```python
from build123d import *

# Parameters (mm, degrees)
BOX006_W                = 2
BOX006_H                = 4.17
BOX006_DEPTH            = 13
ARRAY003_X_COUNT        = 2
ARRAY003_X_PITCH        = 43
ARRAY003_Y_COUNT        = 2
ARRAY003_Y_PITCH        = 27.5
CYLINDER002_R           = 2.1
CYLINDER002_DEPTH       = 2
CYLINDER002_PITCH_ANGLE = 90
ARRAY002_X_COUNT        = 2
ARRAY002_X_PITCH        = 43
ARRAY002_Y_COUNT        = 2
ARRAY002_Y_PITCH        = 27.5
CYLINDER003_R           = 3.25
CYLINDER003_DEPTH       = 2
BOX007_W                = 6.5
BOX007_H                = 36
BOX007_DEPTH            = 2
BOX003_W                = 45
BOX003_H                = 60
BOX003_DEPTH            = 2
BOX005_W                = 2
BOX005_H                = 60
BOX005_DEPTH            = 45
BOX004_W                = 2
BOX004_H                = 60
BOX004_DEPTH            = 45
CUT003_PLACEMENT_ANGLE  = 180


with BuildPart() as array003:
    # Box006 → Box006 (new body)
    with BuildSketch(Plane(origin=(0, 15.6, 37), x_dir=(1, 0, 0), z_dir=(0, 0, 1))):
        with Locations((1, 2.085)):
            Rectangle(BOX006_W, BOX006_H)
    extrude(amount=BOX006_DEPTH)

    # Array003 X: Array003 ×2


with BuildPart() as array003_1:
    add(array003.part)
    with Locations(*[(i * ARRAY003_X_PITCH, 0, 0) for i in range(1, ARRAY003_X_COUNT)]):
        add(array003.part)

    # Array003 Y: Array003 ×2


with BuildPart() as array003_2:
    add(array003_1.part)
    with Locations(*[(0, i * ARRAY003_Y_PITCH, 0) for i in range(1, ARRAY003_Y_COUNT)]):
        add(array003_1.part)


with BuildPart() as fusion003:
    # Cylinder002 → Cylinder002 (new body)
    with BuildSketch(Plane.XY):
        Circle(CYLINDER002_R)
    extrude(amount=CYLINDER002_DEPTH)


with BuildPart() as fusion003_1:
    # Cylinder002 pitch: moved
    add(fusion003.part.rotate(Axis((0, 0, 0), (0, 1, 0)), CYLINDER002_PITCH_ANGLE))


with BuildPart() as fusion003_2:
    # Cylinder002 placement: moved
    add(fusion003_1.part.moved(Location((0, 17.7, 37.1))))

    # Array002 X: Fusion003 ×2


with BuildPart() as fusion003_3:
    add(fusion003_2.part)
    with Locations(*[(i * ARRAY002_X_PITCH, 0, 0) for i in range(1, ARRAY002_X_COUNT)]):
        add(fusion003_2.part)

    # Array002 Y: Fusion003 ×2


with BuildPart() as fusion003_4:
    add(fusion003_3.part)
    with Locations(*[(0, i * ARRAY002_Y_PITCH, 0) for i in range(1, ARRAY002_Y_COUNT)]):
        add(fusion003_3.part)

    # Fusion003: union Array003
    add(array003_2.part)


with BuildPart() as cilindro003:
    # Cylinder003 → Cylinder003 (new body)
    with BuildSketch(Plane(origin=(22.5, 30, 0), x_dir=(1, 0, 0), z_dir=(0, 0, 1))):
        Circle(CYLINDER003_R)
    extrude(amount=CYLINDER003_DEPTH)


with BuildPart() as fusion004:
    # Box007 → Box007 (new body)
    with BuildSketch(Plane(origin=(19.25, 30, 0), x_dir=(1, 0, 0), z_dir=(0, 0, 1))):
        with Locations((3.25, 18)):
            Rectangle(BOX007_W, BOX007_H)
    extrude(amount=BOX007_DEPTH)

    # Fusion002: union Cilindro003
    add(cilindro003.part)

    # Fusion004: union Fusion003
    add(fusion003_4.part)


with BuildPart() as pared_inferior:
    # Box003 → Box003 (new body)
    with BuildSketch(Plane.XY):
        with Locations((22.5, 30)):
            Rectangle(BOX003_W, BOX003_H)
    extrude(amount=BOX003_DEPTH)


with BuildPart() as pared_izquierda:
    # Box005 → Box005 (new body)
    with BuildSketch(Plane(origin=(43, 0, 0), x_dir=(1, 0, 0), z_dir=(0, 0, 1))):
        with Locations((1, 30)):
            Rectangle(BOX005_W, BOX005_H)
    extrude(amount=BOX005_DEPTH)


with BuildPart() as obj1:
    # Box004 → Box004 (new body)
    with BuildSketch(Plane.XY):
        with Locations((1, 30)):
            Rectangle(BOX004_W, BOX004_H)
    extrude(amount=BOX004_DEPTH)

    # Fusion001: union pared inferior, pared izquierda
    add(pared_inferior.part)
    add(pared_izquierda.part)

    # Cut003: cut Fusion004
    add(fusion004.part, mode=Mode.SUBTRACT)


with BuildPart() as obj1_1:
    # Cut003 placement: moved
    add(obj1.part.moved(Location((0, 12, 35))).rotate(Axis((0, 12, 35), (1, 0, 0)), CUT003_PLACEMENT_ANGLE))


solid = obj1_1.part
```
The listing builds one solid part. Answer for the finished solid, in the listing's coordinates (mm). A direction names the side the tool comes from. Round coordinates to 2 decimals unless told otherwise and drop trailing zeros. Loops run counter-clockwise (first coordinate to the right, second up) from the corner with the lowest first, then second, coordinate; pieces in that order, holes last. Notation, with made-up numbers: (-26.75, 40) - (12.25, 40) arc R20 cw to (12.25, 62) - close; hole circle Ø10 at (31, 45). An arc over 180 degrees is marked (long way). Return JSON: item names as keys, results as strings. Group by question number.
1. Each of these flat-tipped pins is pushed along its axis until it touches: P1, Ø12, axis at x = 29, y = -11.5, coming from the -Z side; P2, Ø6, axis at x = 6.5, z = 0, coming from the +Y side. Where does it stop, or does it pass through?
2. The mould has two halves that part along X. Classify faces 1 (the flat face through (17, -18, 35)), 2 (the flat face through (45, -18, 13)), 3 (the flat face through (2, -18, 12)), 4 (the flat face through (19.25, -33, 34)): pulls with the +X half, pulls with the -X half, needs draft (parallel to the pull), parting line crosses it, or undercut.
3. The part is cut by section A-A on y = -30. Determine the outline of the cut face in (x, z), then the cut area to 3 significant figures.
4. The part is cut by section D-D on x = 11. Determine the outline of the cut face in (y, z), then the cut area to 3 significant figures.
5. The part is cut by section C-C on y = -14. Determine the outline of the cut face in (x, z).
6. The part is cut by section B-B on z = 21. Determine the outline of the cut face in (x, y).
7. Which of the six approach directions +Z, -Z, +X, -X, +Y, -Y give full straight-line access (tool end or side, diameter ignored) to faces 5 (the flat face through (1, -7.77, -6)), 6 (the flat face through (22, 12, 34))?
8. Consider probe 1 along X at (y, z) = (-40.5, -3.5); probe 2 along Z at (x, y) = (10, -9). Determine where each line is inside the solid, lowest interval first.
Resolved:
{
 "1": {"P1": "stops at z = 33", "P2": "passes through"},
 "2": {"face 1": "needs draft", "face 2": "pulls with the +X half", "face 3": "undercut", "face 4": "undercut"},
 "3": {"outline": "(0, -10) - (2, -10) - (2, 33) - (19.25, 33) - (19.25, 35) - (0, 35) - close; (25.75, 33) - (43, 33) - (43, -10) - (45, -10) - (45, 35) - (25.75, 35) - close", "area": "249 mm²"},
 "4": {"outline": "(-48, 33) - (12, 33) - (12, 35) - (-48, 35) - close", "area": "120 mm²"},
 "5": {"outline": "(0, -10) - (2, -10) - (2, 33) - (43, 33) - (43, -10) - (45, -10) - (45, 35) - (0, 35) - close"},
 "6": {"outline": "(0, -48) - (2, -48) - (2, 12) - (0, 12) - close; (43, -48) - (45, -48) - (45, 12) - (43, 12) - close"},
 "7": {"face 5": "-Z, +X, -X", "face 6": "+Z, -Z, +X, -X, +Y"},
 "8": {"probe 1": "x = 0 to 2, 43 to 45", "probe 2": "z = 33 to 35"}
}
